Verification items for the finished model (mm, model axes). Face numbers are marked on the shaded views. A direction names the side the tool comes from. Round coordinates to 2 decimals unless told otherwise and drop trailing zeros. Write each loop counter-clockwise with the first axis right and the second up, starting at its lowest first coordinate (ties: lowest second). Pieces come first, ordered by that corner, then holes. Notation, with made-up numbers: M 8,26 L 41,26 A17 cw 41,38 Z; hole C 53,58.25 d3. An arc over 180 degrees is marked long. Write each question's results on one line, items separated by ' | '.
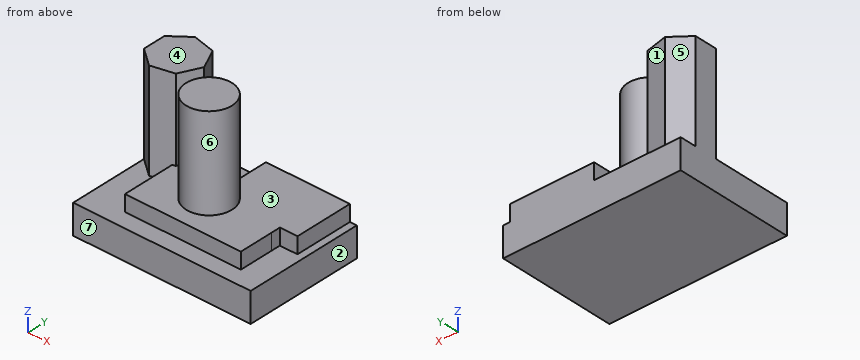
from build123d import *

# Parameters (mm, degrees)
F0_W     = 76.2
F0_H     = 50.8
F1_DEPTH = 12.7
F2_W     = 49.7612692416
F2_H     = 14.612480998
F2_W_2   = 28.4890644252
F2_H_2   = 11.0769122839
F3_DEPTH = 6.9243321195
F4_R     = 9.8381563478
F5_DEPTH = 39.9880222976
F7_DEPTH = 42.3764139414


with BuildPart() as f1:
    # F0 (on Top) → F1 (new body)
    with BuildSketch(Plane.XY):
        with Locations((-38.1, -188.4133778646)):
            Rectangle(F0_W, F0_H)
    extrude(amount=-F1_DEPTH)

    # F2 (on face) → F3 (join)
    with BuildSketch(Plane.XY):
        with Locations((-35.398973152, -199.4379386306)):
            Rectangle(F2_W, F2_H)
        Polygon((-60.2796077728, -177.0403236151), (-60.2796077728, -192.1316981316), (-10.5183385313, -192.1316981316), (-10.5183385313, -188.117235899), (-39.0074029565, -188.117235899), (-39.0074029565, -177.0403236151), align=None)
        with Locations((-24.7628707439, -182.578779757)):
            Rectangle(F2_W_2, F2_H_2)
        Polygon((-10.5183385313, -177.0403236151), (-10.5183385313, -188.117235899), (-2.9622917064, -188.117235899), (-2.9622917064, -163.0133778646), (-39.0074029565, -163.0133778646), (-39.0074029565, -177.0403236151), align=None)
    extrude(amount=F3_DEPTH)

    # F4 (on face) → F5 (join)
    with BuildSketch(Plane.XY.offset(6.9243321195)):
        with Locations((-38.5907627642, -190.6945705414)):
            Circle(F4_R)
    extrude(amount=F5_DEPTH)

    # F6 (on face) → F7 (join)
    with BuildSketch(Plane.XY):
        Polygon((-76.2, -170.1574557203), (-76.2, -179.9530751329), (-68.5414763529, -186.0605439396), (-58.9914535705, -183.8808135592), (-54.7412935927, -175.0552654266), (-58.9914535705, -166.229717294), (-68.5414763529, -164.0499869137), align=None)
    extrude(amount=F7_DEPTH)


solid = f1.part
1) Sectioned sample at C-C, the plane x = -25.5. Record the cut outline in (y, z), and give its area (3 significant figures).
Calculated:
outline: M -213.81,-12.7 L -163.01,-12.7 L -163.01,6.92 L -206.74,6.92 L -206.74,0 L -213.81,0 Z | area: 948 mm²
2) Sectioned sample at B-B, the plane z = 23. Record the cut outline in (x, y), and give its area (3 significant figures).
Calculated:
outline: M -76.2,-179.95 L -68.54,-186.06 L -58.99,-183.88 L -54.74,-175.06 L -58.99,-166.23 L -68.54,-164.05 L -76.2,-170.16 Z; C -38.59,-190.69 d19.68 | area: 653 mm²
3) Sectioned sample at A-A, the plane y = -205. Record the cut outline in (x, z), and give its area (3 significant figures).
Calculated:
outline: M -76.2,-12.7 L 0,-12.7 L 0,0 L -10.52,0 L -10.52,6.92 L -60.28,6.92 L -60.28,0 L -76.2,0 Z | area: 1,310 mm²
4) Access from +Z, -Z, +X, -X, +Y, -Y to the whole of each face (thin tool, end or side, straight path). Record for the marked faces 1, 2, 3 and 4.
Calculated:
face 1: +Z, +Y | face 2: +Z, -Z, +X, +Y, -Y | face 3: +Z | face 4: +Z, -X, +Y, -Y
5) Material ranges on line 1 (Z direction, x = -8.5, y = -191); line 2 (Z direction, x = -16.5, y = -203); line 3 (Y direction, x = -8, z = 1), recorded low to high. Write a range as [from, to].
Calculated:
line 1: z = [-12.7, 0] | line 2: z = [-12.7, 6.92] | line 3: y = [-188.12, -163.01]
6) Draft check along X on the marked faces 5, 6 and 7. Enter one of: pulls with the +X half, pulls with the -X half, needs draft (parallel to the pull), parting line crosses it, or undercut.
Calculated:
face 5: pulls with the -X half | face 6: undercut | face 7: needs draft
7) Depth check by flat-ended pin: P1, Ø5.5, axis at x = -5.5, z = 5, coming from the -Y side; P2, Ø4, axis at x = -59, y = -169.5, coming from the +Z side; P3, Ø3, axis at y = -190, z = 5, coming from the +X side. Enter the tip coordinate at first touch or a pass-through.
Calculated:
P1: stops at y = -188.12 | P2: stops at z = 42.38 | P3: stops at x = -10.52
8) Sectioned sample at D-D, the plane z = 3.5. Record the cut outline in (x, y), and give its area (3 significant figures).
Calculated:
outline: M -76.2,-179.95 L -68.54,-186.06 L -60.28,-184.17 L -60.28,-206.74 L -10.52,-206.74 L -10.52,-188.12 L -2.96,-188.12 L -2.96,-163.01 L -39.01,-163.01 L -39.01,-177.04 L -55.7,-177.04 L -54.74,-175.06 L -58.99,-166.23 L -68.54,-164.05 L -76.2,-170.16 Z | area: 2,400 mm²
